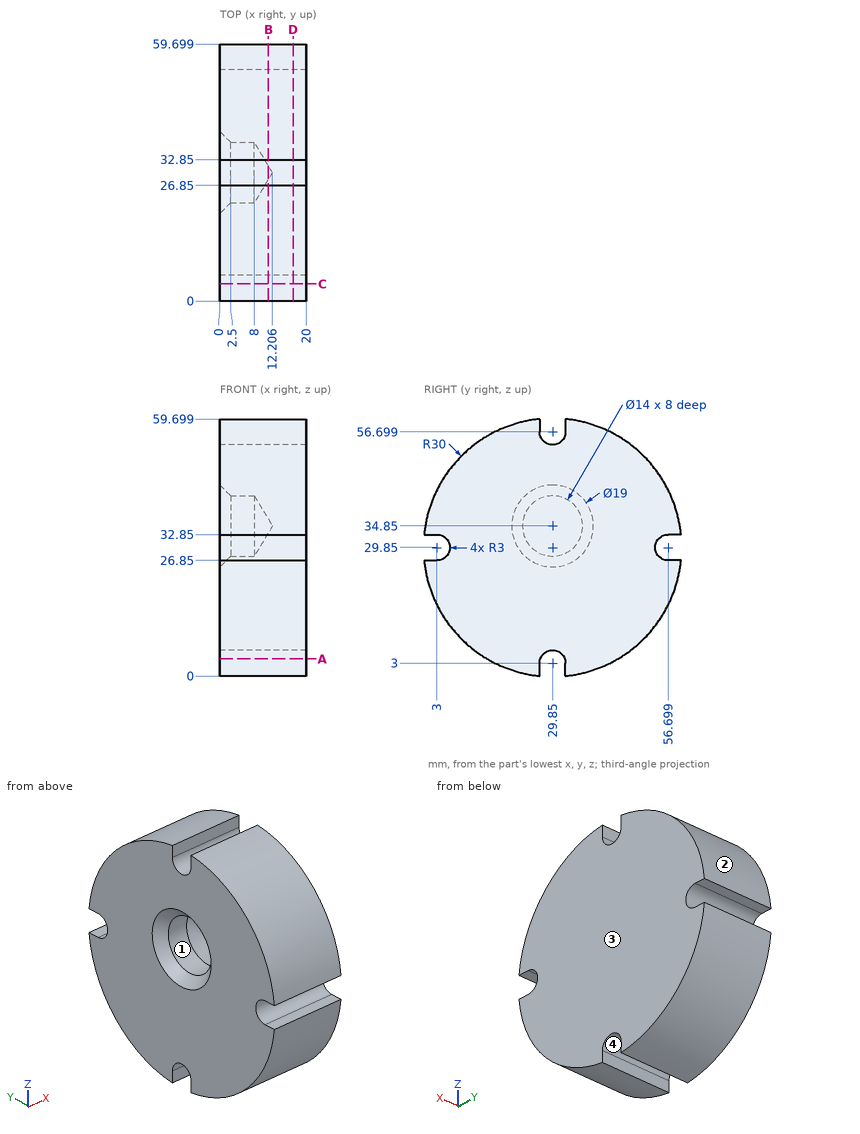
Could you check a few things on this drawing? It's one solid part, dimensions in mm from its lowest x, y, z. Coordinates: 2 decimals unless noted, no trailing zeros. Write each loop counter-clockwise with the first axis right and the second up, starting at its lowest first coordinate (ties: lowest second). Pieces come first, ordered by that corner, then holes. Notation, with made-up numbers: (88, -40) - (104, -40) arc R26 cw to (104, -13) - close; hole circle Ø3 at (-11, 33.5). An arc over 180 degrees is marked (long way). Return JSON: item names as keys, results as strings. Group by question number.
Item 1: We'd pull the mould along Y, two halves only. Please class the marked faces 1, 2, 3 and 4: pulls with the +Y half, pulls with the -Y half, needs draft (parallel to the pull), parting line crosses it, or undercut.
Item 2: If we section it at D-D (x = 17): Write out the boundary of the cut face in (y, z).
Item 3: Please list where these lines run through material, in increasing order: probe 1 along Y at (x, z) = (4.5, 32) (1 decimal); probe 2 along Y at (x, z) = (18.25, 56.5) (1 decimal); probe 3 along Y at (x, z) = (3.5, 20.5) (1 decimal).
Item 4: If we section it at A-A (z = 4): Write out the boundary of the cut face in (x, y) (1 decimal), then the cut area to 3 significant figures.
Item 5: I'm going to push flat-ended pins straight in: pin 1 Ø5 at (x, z) = (9, 13) entering from +Y (1 decimal); pin 2 Ø3.5 at (x, z) = (7, 1) entering from -Y; pin 3 Ø4 at (x, y) = (6.5, 26.5) entering from -Z; pin 4 Ø8 at (x, y) = (4, 10.5) entering from +Z (1 decimal). Where does each tip first touch, or does it pass through?
Item 6: If we section it at B-B (x = 11.25): Write out the boundary of the cut face in (y, z), then the cut area to 3 significant figures.
Return value:
{
 "1": {"face 1": "undercut", "face 2": "pulls with the +Y half", "face 3": "needs draft", "face 4": "undercut"},
 "2": {"outline": "(0, 26.85) arc R30 ccw to (26.85, 0) - (26.85, 3) arc R3 cw to (32.85, 3) - (32.85, 0) arc R30 ccw to (59.7, 26.85) - (56.7, 26.85) arc R3 cw to (56.7, 32.85) - (59.7, 32.85) arc R30 ccw to (32.85, 59.7) - (32.85, 56.7) arc R3 cw to (26.85, 56.7) - (26.85, 59.7) arc R30 ccw to (0, 32.85) - (3, 32.85) arc R3 cw to (3, 26.85) - close"},
 "3": {"probe 1": "y = 5.1 to 23.5, 36.2 to 54.6", "probe 2": "y = 16.1 to 26.9, 32.8 to 43.6", "probe 3": "y = 1.3 to 58.4"},
 "4": {"outline": "(0, 14.6) - (20, 14.6) - (20, 27) - (0, 27) - close; (0, 32.7) - (20, 32.7) - (20, 45.1) - (0, 45.1) - close", "area": "496 mm^2"},
 "5": {"pin 1": "stops at y = 56.2", "pin 2": "stops at y = 16.98", "pin 3": "stops at z = 0", "pin 4": "stops at z = 55.6"},
 "6": {"outline": "(0, 26.85) arc R30 ccw to (26.85, 0) - (26.85, 3) arc R3 cw to (32.85, 3) - (32.85, 0) arc R30 ccw to (59.7, 26.85) - (56.7, 26.85) arc R3 cw to (56.7, 32.85) - (59.7, 32.85) arc R30 ccw to (32.85, 59.7) - (32.85, 56.7) arc R3 cw to (26.85, 56.7) - (26.85, 59.7) arc R30 ccw to (0, 32.85) - (3, 32.85) arc R3 cw to (3, 26.85) - close; hole circle Ø3.18 at (29.85, 34.85)", "area": "2,690 mm^2"}
}
